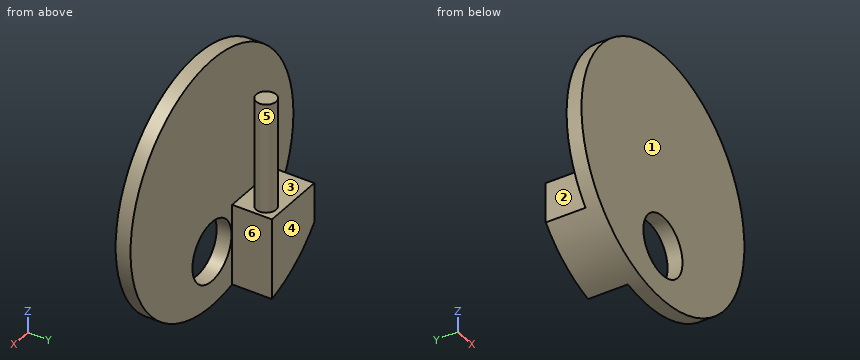
from build123d import *

# Parameters (mm, degrees)
SKETCH1_R                = 12.5
SKETCH1_R_2              = 3
BOSS_EXTRUDE1_DEPTH      = 1.5
SKETCH3_R                = 1
BOSS_EXTRUDE3_DEPTH      = 11
BOSS_EXTRUDE4_REACH      = 23.296
BOSS_EXTRUDE4_END_RADIUS = 12.5
SKETCH5_W                = 6.5
SKETCH5_H                = 4


with BuildPart() as part:
    # Sketch1 → Boss-Extrude1 (new body)
    with BuildSketch(Plane(origin=(0, 0, 0), x_dir=(1, 0, 0), z_dir=(0, 1, 0))):
        with Locations(Location((0, 0, 0), (0, 0, 270))):
            Circle(SKETCH1_R)
        with Locations(Location((0, 7, 0), (0, 0, 270))):
            Circle(SKETCH1_R_2, mode=Mode.SUBTRACT)
    extrude(amount=BOSS_EXTRUDE1_DEPTH)



with BuildPart() as body_2:
    # Sketch3 → Boss-Extrude3 (new body)
    with BuildSketch(Plane.XY.offset(-4)):
        with Locations((-4.5, 4)):
            Circle(SKETCH3_R)
    extrude(amount=BOSS_EXTRUDE3_DEPTH)


with BuildPart() as part_1:
    add(part.part)

    add(body_2.part)  # Boss-Extrude4 merges body 2
    # Boss-Extrude4: up to this cylinder (the profile starts inside it)
    boss_extrude4_end = Plane(origin=(0, 3.5, 0), z_dir=(0, -1, 0)) * Cylinder(BOSS_EXTRUDE4_END_RADIUS, 72.592, mode=Mode.PRIVATE)
    # Sketch5 → Boss-Extrude4 (add, up to the surface)
    with BuildSketch(Plane.XY.offset(-4), mode=Mode.PRIVATE) as boss_extrude4_sk1:
        with Locations((-6.35, 3.5)):
            Rectangle(SKETCH5_W, SKETCH5_H)
    boss_extrude4_tool1 = extrude(boss_extrude4_sk1.sketch, amount=-BOSS_EXTRUDE4_REACH, mode=Mode.PRIVATE) & boss_extrude4_end
    add(boss_extrude4_tool1.solids().sort_by_distance((-6.35, 3.5, -4))[0])


solid = part_1.part
Design review of the part built by this model. Coordinates are the model's own, in mm. Face numbers are marked on the shaded views. A direction names the side the tool comes from. Coordinates: 2 decimals unless noted, no trailing zeros. Loops run counter-clockwise (first coordinate to the right, second up) from the corner with the lowest first, then second, coordinate; pieces in that order, holes last. Notation, with made-up numbers: M 9.25,39.5 L 28.25,39.5 A17 ccw 28.25,63.5 Z; hole C -38,-28 d8. An arc over 180 degrees is marked long. Use one line per item in the form item = value.
(1) Clearance check with flat-ended pins moving along their axes: P1, Ø3, axis at x = -3, z = -5, coming from the +Y side; P2, Ø1.5, axis at x = -9.5, z = 9.5, coming from the +Y side; P3, Ø1.2, axis at x = -6.5, y = 3, coming from the +Z side; P4, Ø3, axis at x = -6.5, y = 5, coming from the +Z side. State where each tip first meets the part, or that it passes through.
Return value:
P1 = 5.5
P2 = through
P3 = -4
P4 = 7
(2) Consider section B-B (x = 0). Write out the cut boundary in (y, z).
Return value:
outline = M 0,-12.5 L 1.5,-12.5 L 1.5,-10 L 0,-10 Z; M 0,-4 L 1.5,-4 L 1.5,12.5 L 0,12.5 Z
(3) Consider section D-D (x = -4.75). Write out the cut boundary in (y, z), and give its area (3 significant figures).
Return value:
outline = M 0,-11.56 L 5.5,-11.56 L 5.5,-4 L 4.97,-4 L 4.97,7 L 3.03,7 L 3.03,-4 L 1.5,-4 L 1.5,11.56 L 0,11.56 Z
area = 86.2 mm2
(4) Consider section A-A (z = 0.5). Write out the cut boundary in (x, y), and give its area (3 significant figures).
Return value:
outline = M -12.49,0 L 12.49,0 L 12.49,1.5 L -12.49,1.5 Z; C -4.5,4 d2
area = 40.6 mm2
(5) Draft analysis for pull direction Y (two halves, no side actions). For the marked faces 1, 2 and 3, state which applies: pulls with the +Y half, pulls with the -Y half, needs draft (parallel to the pull), parting line crosses it, or undercut.
Return value:
face_1 = pulls with the -Y half
face_2 = needs draft
face_3 = undercut
(6) For the marked faces 4, 5 and 6, list the 3-axis set-ups (+Z, -Z, +X, -X, +Y, -Y) from which the entire face can be reached by the end or side of a thin tool; tool diameter is ignored.
Return value:
face_4 = +Z, -Z, +X, -X, +Y
face_5 = +Z
face_6 = +Z, -Z, +X, +Y
(7) Consider section C-C (y = 4). Write out the cut boundary in (x, z).
Return value:
outline = M -9.6,-8.01 A12.5 ccw -3.1,-12.11 L -3.1,-4 L -3.5,-4 L -3.5,7 L -5.5,7 L -5.5,-4 L -9.6,-4 Z
(8) For line 1 along Y through (x, z) = (-8, 1.75); line 2 along X through (y, z) = (1.15, -7); line 3 along X through (y, z) = (2.1, -5.25), list the stretches that pass through material, from the lowest coordinate up. Write a range as from..to.
Return value:
line_1 = 0..1.5
line_2 = -10.36..-3, 3..10.36
line_3 = -9.6..-3.1
